Part print with two shaded views. Sizes in mm from the minimum x, y, z corner. A direction names the side the tool comes from. Round coordinates to 2 decimals unless told otherwise and drop trailing zeros. Loops run counter-clockwise (first coordinate to the right, second up) from the corner with the lowest first, then second, coordinate; pieces in that order, holes last. Notation, with made-up numbers: (-9, 13.25) - (6, 13.25) arc R27 ccw to (6, 35.25) - close; hole circle Ø6 at (64.5, 69.5). An arc over 180 degrees is marked (long way). One line per question, with ' | ' between items.
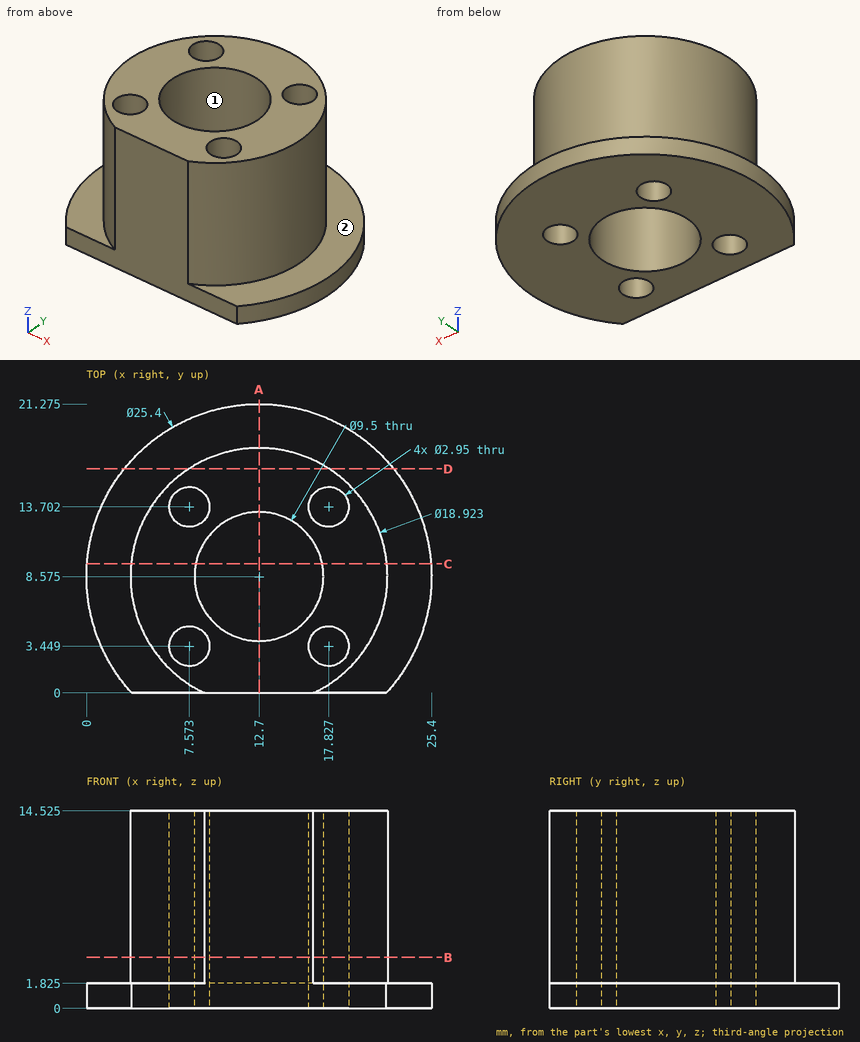
(1) Cut at B-B, the plane z = 3.75. State how many separate pieces and enclosed holes the cut face has, then the cut area to 3 significant figures.
Results found:
separate pieces: 1 | enclosed holes: 5 | area: 178 mm²
(2) Cut at A-A, the plane x = 12.7. Write the cut outline in (y, z) (1 decimal), then the cut area to 3 significant figures.
Results found:
outline: (0, 0) - (3.8, 0) - (3.8, 14.5) - (0, 14.5) - close; (13.3, 0) - (21.3, 0) - (21.3, 1.8) - (18, 1.8) - (18, 14.5) - (13.3, 14.5) - close | area: 130 mm²
(3) Tool access for the marked faces 1 and 2: list every direction of +Z, -Z, +X, -X, +Y, -Y with a clear straight run to the whole face (end or side of a thin tool).
Results found:
face 1: +Z, -Z | face 2: +Z
(4) Cut at C-C, the plane y = 9.5. Write the cut outline in (x, z) (1 decimal), then the cut area to 3 significant figures.
Results found:
outline: (0, 0) - (8, 0) - (8, 14.5) - (3.3, 14.5) - (3.3, 1.8) - (0, 1.8) - close; (17.4, 0) - (25.4, 0) - (25.4, 1.8) - (22.1, 1.8) - (22.1, 14.5) - (17.4, 14.5) - close | area: 150 mm²
(5) Drop flat-ended pins along their axis: P1, Ø4, axis at y = 6.5, z = 4.5, coming from the +X side; P2, Ø5, axis at x = 5.5, z = 6.5, coming from the -Y side. Give the stop position or say it passes through.
Results found:
P1: stops at x = 22.16 | P2: stops at y = 0.36
(6) Probe L1, parallel to X at y = 3.75, z = 10.5; L2, parallel to Z at x = 20, y = 16.75 (1 decimal); L3, parallel to X at y = 6.5, z = 12.25. List the from-to ranges inside material, lowest first.
Results found:
L1: x = 4.56 to 6.13, 9.02 to 16.38, 19.27 to 20.84 | L2: z = 0 to 1.8 | L3: x = 3.47 to 8.43, 16.97 to 21.93
(7) Cut at D-D, the plane y = 16.5. Write the cut outline in (x, z) (1 decimal).
Results found:
outline: (2.8, 0) - (22.6, 0) - (22.6, 1.8) - (17.9, 1.8) - (17.9, 14.5) - (7.5, 14.5) - (7.5, 1.8) - (2.8, 1.8) - close
